```python
from build123d import *

# Parameters (mm, degrees)
BOSS_EXTRUDE1_DEPTH = 6.35
SKETCH2_R           = 1.59
CUT_EXTRUDE1_DEPTH  = 1.57
SKETCH3_R           = 1.59
CUT_EXTRUDE2_DEPTH  = 1.57
FILLET1_R           = 1


with BuildPart() as part:
    # Sketch1 → Boss-Extrude1 (new body)
    with BuildSketch(Plane.XY):
        Polygon((0, 8.71), (1.57, 8.71), (1.57, 1.57), (9.53, 1.57), (9.53, 0), (0, 0), align=None)
    extrude(amount=BOSS_EXTRUDE1_DEPTH)

    # Sketch2 → Cut-Extrude1 (cut)
    with BuildSketch(Plane(origin=(0, 1.57, 0), x_dir=(1, 0, 0), z_dir=(0, 1, 0))):
        with Locations(Location((6.35, -3.175, 0), (0, 0, 270))):
            Circle(SKETCH2_R)
    extrude(amount=-CUT_EXTRUDE1_DEPTH, mode=Mode.SUBTRACT)

    # Sketch3 → Cut-Extrude2 (cut)
    with BuildSketch(Plane(origin=(1.57, 0, 0), x_dir=(0, 0, -1), z_dir=(1, 0, 0))):
        with Locations(Location((-3.175, 5.16, 0), (0, 0, 90))):
            Circle(SKETCH3_R)
    extrude(amount=-CUT_EXTRUDE2_DEPTH, mode=Mode.SUBTRACT)

    # Fillet1
    fillet1_edges = [part.edges().sort_by_distance(p)[0] for p in [
        (9.53, 1.57, 3.175),
    ]]
    fillet(fillet1_edges, radius=FILLET1_R)


solid = part.part
```
The listing builds one solid part. Answer for the finished solid, in the listing's coordinates (mm). A direction names the side the tool comes from. Give positions to 0.01 mm unless a question says otherwise; leave off trailing zeros. Loops run counter-clockwise (first coordinate to the right, second up) from the corner with the lowest first, then second, coordinate; pieces in that order, holes last. Notation, with made-up numbers: (-0.75, 15.5) - (13.25, 15.5) arc R23 cw to (13.25, 35.5) - close; hole circle Ø9 at (15, -5). An arc over 180 degrees is marked (long way). Return JSON: item names as keys, results as strings. Group by question number.
1. Straight lines are drawn through the part: line 1 (Z direction, x = 0.3, y = 5.16) (3 decimals); line 2 (Y direction, x = 3, z = 5). For each, find the intervals that lie inside material, in ascending order. Write a range as [from, to].
2. Determine the mould class of faces 1 (the flat face through (0, 3, 3)), 2 (the cylindrical face through (7.42, 0.8, 2)), 3 (the flat face through (1, 8.71, 3)) for opening direction X: pulls with the +X half, pulls with the -X half, needs draft (parallel to the pull), parting line crosses it, or undercut.
3. Find section A-A (x = 6.35). Write down the section's boundary in (y, z) (3 decimals), then the cut area to 3 significant figures.
4. Find section D-D (z = 5). Write down the section's boundary in (x, y).
5. Given pin 1 Ø3 at (x, z) = (5, 4.5) entering from +Y; pin 2 Ø2 at (y, z) = (7, 4.5) entering from +X, each flat-ended and moving along its own axis, determine where each tip first touches the part or whether it passes through.
6. Find section C-C (z = 3.75). Write down the section's boundary in (x, y).
7. Which of the six approach directions +Z, -Z, +X, -X, +Y, -Y give full straight-line access (tool end or side, diameter ignored) to faces 4 (the flat face through (1.57, 7, 3)), 5 (the flat face through (3, 1, 0))?
Verdict:
{
 "1": {"line 1": "z = [0, 1.585], [4.765, 6.35]", "line 2": "y = [0, 1.57]"},
 "2": {"face 1": "pulls with the -X half", "face 2": "undercut", "face 3": "needs draft"},
 "3": {"outline": "(0, 0) - (1.57, 0) - (1.57, 1.585) - (0, 1.585) - close; (0, 4.765) - (1.57, 4.765) - (1.57, 6.35) - (0, 6.35) - close", "area": "4.98 mm^2"},
 "4": {"outline": "(0, 0) - (9.53, 0) - (9.53, 0.57) arc R1 ccw to (8.53, 1.57) - (1.57, 1.57) - (1.57, 8.71) - (0, 8.71) - close"},
 "5": {"pin 1": "stops at y = 1.57", "pin 2": "stops at x = 1.57"},
 "6": {"outline": "(0, 0) - (4.87, 0) - (4.87, 1.57) - (1.57, 1.57) - (1.57, 3.68) - (0, 3.68) - close; (0, 6.64) - (1.57, 6.64) - (1.57, 8.71) - (0, 8.71) - close; (7.83, 0) - (9.53, 0) - (9.53, 0.57) arc R1 ccw to (8.53, 1.57) - (7.83, 1.57) - close"},
 "7": {"face 4": "+Z, -Z, +X, +Y", "face 5": "-Z, +X, -X, +Y, -Y"}
}
